Can you work these out from the model? Positions are in its coordinate system, mm. A direction names the side the tool comes from. Give positions to 0.01 mm unless a question says otherwise; leave off trailing zeros. Order: outer loops, then holes, each group sorted by start corner. A loop starts at its lowest first (then second) coordinate and runs counter-clockwise, first axis right, second up.
Item 1: I want a section at D-D, the plane x = -5.25. Write out the boundary of the cut face in (y, z).
Item 2: I want a section at A-A, the plane x = 0. Write out the boundary of the cut face in (y, z).
Item 3: I want a section at C-C, the plane z = 10. Write out the boundary of the cut face in (x, y) (1 decimal).
Item 4: If we mould it in two halves opening along Y, with no side actions, what happens to faces 1 (the flat face through (3.4, 0.1, 8.588)), 2 (the cylindrical face through (-2.08, 9.36, -3.25)), 3 (the flat face through (2, 6.3, 0))? For each: +Y half, -Y half, draft (parallel to the pull), parting line (faces both ways), or undercut.
Item 5: If I drill on line 1 along Z through (x, y) = (1.25, 8); line 2 along X through (y, z) = (0, -4.5); line 3 along Z through (x, y) = (-4, -5.5), over which ranges is the centre line in solid material (lowest first)?
Item 6: I'm going to push flat-ended pins straight in: pin 1 Ø6 at (y, z) = (3, 1) entering from +X; pin 2 Ø4 at (x, y) = (-3, 2) entering from +Z; pin 3 Ø1.5 at (x, z) = (-6.5, -4) entering from -Y. Where does each tip first touch, or does it pass through?
Item 7: Which directions (+Z, -Z, +X, -X, +Y, -Y) give clear straight access to the entire face, cutting with the end or side of a thin tool? Please do faces 4 (the cylindrical face through (-1.38, -6.2, 3.45)), 5 (the cylindrical face through (-1.73, -7.81, 11.05)), 6 (the cylindrical face through (-1.73, 7.81, -4.05)).
```python
from build123d import *

# Parameters (mm, degrees)
F0_R     = 6.35
F0_R_2   = 2.89687
F1_DEPTH = 7
F2_R     = 9.587497
F2_R_2   = 2.89687
F3_DEPTH = 1.5875
F4_R     = 9.587497
F4_R_2   = 8
F5_DEPTH = 5
F6_R     = 9.587497
F6_R_2   = 2.89687
F7_DEPTH = 1.5875
F8_R     = 9.587497
F8_R_2   = 8
F9_DEPTH = 5


with BuildPart() as f1:
    # F0 (on Top) → F1 (new body)
    with BuildSketch(Plane.XY):
        Circle(F0_R)
        Circle(F0_R_2, mode=Mode.SUBTRACT)
    extrude(amount=F1_DEPTH)

    # F2 (on face) → F3 (join)
    with BuildSketch(Plane.XY.offset(7)):
        Circle(F2_R)
        Circle(F2_R_2, mode=Mode.SUBTRACT)
    extrude(amount=F3_DEPTH)



with BuildPart() as f5:
    # F4 (on face) → F5 (new body)
    with BuildSketch(Plane(origin=(0, 0, -1.5875), x_dir=(1, 0, 0), z_dir=(0, 0, -1))):
        Circle(F4_R)
        Circle(F4_R_2, mode=Mode.SUBTRACT)
    extrude(amount=F5_DEPTH)


with BuildPart() as f1_1:
    add(f1.part)

    add(f5.part)  # F7 merges F5
    # F6 (on face) → F7 (join)
    with BuildSketch(Plane(origin=(0, 0, 0), x_dir=(1, 0, 0), z_dir=(0, 0, -1))):
        Circle(F6_R)
        Circle(F6_R_2, mode=Mode.SUBTRACT)
    extrude(amount=F7_DEPTH)

    # F8 (on face) → F9 (join)
    with BuildSketch(Plane.XY.offset(8.5875)):
        Circle(F8_R)
        Circle(F8_R_2, mode=Mode.SUBTRACT)
    extrude(amount=F9_DEPTH)


solid = f1_1.part
```
Results list:
1. outline: (-8.02, -6.59) - (-6.04, -6.59) - (-6.04, -1.59) - (6.04, -1.59) - (6.04, -6.59) - (8.02, -6.59) - (8.02, 0) - (3.57, 0) - (3.57, 7) - (8.02, 7) - (8.02, 13.59) - (6.04, 13.59) - (6.04, 8.59) - (-6.04, 8.59) - (-6.04, 13.59) - (-8.02, 13.59) - (-8.02, 7) - (-3.57, 7) - (-3.57, 0) - (-8.02, 0) - close
2. outline: (-9.59, -6.59) - (-8, -6.59) - (-8, -1.59) - (-2.9, -1.59) - (-2.9, 8.59) - (-8, 8.59) - (-8, 13.59) - (-9.59, 13.59) - (-9.59, 7) - (-6.35, 7) - (-6.35, 0) - (-9.59, 0) - close; (2.9, -1.59) - (8, -1.59) - (8, -6.59) - (9.59, -6.59) - (9.59, 0) - (6.35, 0) - (6.35, 7) - (9.59, 7) - (9.59, 13.59) - (8, 13.59) - (8, 8.59) - (2.9, 8.59) - close
3. outline: circle Ø19.2 at (0, 0); hole circle Ø16 at (0, 0)
4. face 1: undercut
4. face 2: parting line
4. face 3: draft
5. line 1: z = -6.59 to 0, 7 to 13.59
5. line 2: x = -9.59 to -8, 8 to 9.59
5. line 3: z = -1.59 to 0, 7 to 8.59
6. pin 1: stops at x = 9.59
6. pin 2: stops at z = 8.59
6. pin 3: stops at y = -7.67
7. face 4: none
7. face 5: +Z
7. face 6: -Z
